Verification items for the finished model (mm, model axes). Face numbers are marked on the shaded views. A direction names the side the tool comes from. Round coordinates to 2 decimals unless told otherwise and drop trailing zeros. Write each loop counter-clockwise with the first axis right and the second up, starting at its lowest first coordinate (ties: lowest second). Pieces come first, ordered by that corner, then holes. Notation, with made-up numbers: (-25, 1.5) -> (-5, 1.5) arc R24 cw to (-5, 24.5) -> close; hole circle Ø9 at (-8, 26). An arc over 180 degrees is marked (long way). Answer as a JSON object with one key per item and string values. Group by question number.
(1) Sectioned sample at D-D on z = -8.5. Record the cut outline in (x, y).
(2) Set-up check for the marked faces 1 and 2: record each of +Z, -Z, +X, -X, +Y, -Y from which the full face is reachable in a straight line by a thin tool's end or side.
(3) Gauge pin test, flat ends, axial feed: pin 1 Ø2.5 at (x, z) = (0, -17) entering from -Y; pin 2 Ø4.5 at (x, z) = (-14.72, -8.5) entering from -Y; pin 3 Ø1.5 at (x, y) = (52.5, 1.5) entering from -Z; pin 4 Ø0.9 at (x, y) = (-53, 1.5) entering from +Z. Record the tip position at first contact, or that the pin passes through.
(4) Scan lines: L1, parallel to Z at x = -53.85, y = -1.05; L2, parallel to Z at x = 15.5, y = -1; L3, parallel to X at y = -4.6, z = 52.5. Record each from-to range of solid material in increasing order. Write a range as from..to.
(5) Sectioned sample at B-B on x = 53.85. Record the cut outline in (y, z).
(6) Sectioned sample at A-A on z = 52.5. Record the cut outline in (x, y), and give its area (3 significant figures).
(7) Sectioned sample at C-C on x = 11.5. Record the cut outline in (y, z), and give its area (3 significant figures).
```python
from build123d import *

# Parameters (mm, degrees)
SKETCH_1_W                  = 123
SKETCH_1_H                  = 130
EXTRUDE_1_DEPTH             = 5
EXTRUDE_2_DEPTH             = 3
HOLE_WIZARD_13_0_13_1_D     = 13
HOLE_WIZARD_13_0_13_1_DEPTH = 6
HOLE_WIZARD_2_5_2_5_1_D     = 2.5
HOLE_WIZARD_2_5_2_5_1_DEPTH = 5
HOLE_WIZARD_3_3_3_3_1_D     = 3.3
HOLE_WIZARD_3_3_3_3_1_DEPTH = 6
HOLE_WIZARD_1_D             = 5.2
HOLE_WIZARD_1_DEPTH         = 8
HOLE_WIZARD_1_CBORE_D       = 11
HOLE_WIZARD_1_CBORE_DEPTH   = 1
CHAMFER_1_SIZE              = 0.2
FILLET_1_R                  = 0.5
FILLET_2_R                  = 1


with BuildPart() as part:
    # 草图1 → 凸台-拉伸1 (new body)
    with BuildSketch(Plane(origin=(0, 0, 0), x_dir=(1, 0, 0), z_dir=(0, 1, 0))):
        Rectangle(SKETCH_1_W, SKETCH_1_H)
    extrude(amount=-EXTRUDE_1_DEPTH)

    # 草图2 → 凸台-拉伸2 (add)
    with BuildSketch(Plane(origin=(0, 0, 0), x_dir=(-1, 0, 0), z_dir=(0, 1, 0))):
        with BuildLine():
            Line((46.2, -45), (46.2, -60))
            Line((46.2, -60), (-46.2, -60))
            Line((-46.2, -60), (-46.2, -45))
            ThreePointArc((-46.2, -45), (-46.7, -44.5), (-47.2, -45))
            Line((-47.2, -45), (-60, -45))
            Line((-60, -45), (-60, 45))
            Line((-60, 45), (-47.2, 45))
            ThreePointArc((-47.2, 45), (-46.7, 44.5), (-46.2, 45))
            Line((-46.2, 45), (-46.2, 60))
            Line((-46.2, 60), (46.2, 60))
            Line((46.2, 60), (46.2, 45))
            ThreePointArc((46.2, 45), (46.7, 44.5), (47.2, 45))
            Line((47.2, 45), (60, 45))
            Line((60, 45), (60, -45))
            Line((60, -45), (47.2, -45))
            ThreePointArc((47.2, -45), (46.7, -44.5), (46.2, -45))
        make_face()
    extrude(amount=EXTRUDE_2_DEPTH)

    # Ø13.0 (13) 直径孔1
    with Locations(Plane(origin=(0, -5, 0), x_dir=(-1, 0, 0), z_dir=(0, -1, 0))):
        with Locations((0, 0)):
            Hole(HOLE_WIZARD_13_0_13_1_D / 2, depth=HOLE_WIZARD_13_0_13_1_DEPTH)

    # Ø2.5 (2.5) 直径孔1
    with Locations(Plane(origin=(0, 3, 0), x_dir=(1, 0, 0), z_dir=(0, 1, 0))):
        with Locations((-56.780566421, -41.855346711), (-11.041427483, 41.956342393), (-56.907566675, 41.837820676), (-11.168427737, -41.75982474)):
            Hole(HOLE_WIZARD_2_5_2_5_1_D / 2, depth=HOLE_WIZARD_2_5_2_5_1_DEPTH)

    # Ø3.3 (3.3) 直径孔1
    with Locations(Plane(origin=(0, -5, 0), x_dir=(-1, 0, 0), z_dir=(0, -1, 0))):
        with Locations((-14.722431864, -8.5), (-14.722431864, 8.5), (0, 17), (14.722431864, 8.5), (14.722431864, -8.5), (0, -17)):
            Hole(HOLE_WIZARD_3_3_3_3_1_D / 2, depth=HOLE_WIZARD_3_3_3_3_1_DEPTH)

    # 孔1
    with Locations(Plane(origin=(0, -5, 0), x_dir=(-1, 0, 0), z_dir=(0, -1, 0))):
        with Locations((53.85, 52.5), (-53.85, -52.5), (53.85, -52.5), (-53.85, 52.5)):
            CounterBoreHole(HOLE_WIZARD_1_D / 2, HOLE_WIZARD_1_CBORE_D / 2, HOLE_WIZARD_1_CBORE_DEPTH, depth=HOLE_WIZARD_1_DEPTH)

    # 倒角1
    chamfer_1_edges = [part.edges().sort_by_distance(p)[0] for p in [
        (0, -5, 65),
        (0, -5, -65),
    ]]
    chamfer(chamfer_1_edges, length=CHAMFER_1_SIZE)

    # 圆角1
    fillet_1_edges = [part.edges().sort_by_distance(p)[0] for p in [
        (-60, 1.5, -45),
        (-60, 1.5, 45),
        (-46.2, 1.5, 60),
        (46.2, 1.5, 60),
        (60, 1.5, 45),
        (60, 1.5, -45),
        (46.2, 1.5, -60),
        (-46.2, 1.5, -60),
    ]]
    fillet(fillet_1_edges, radius=FILLET_1_R)

    # 圆角2
    fillet_2_edges = [part.edges().sort_by_distance(p)[0] for p in [
        (-47.2, 1.5, -45),
        (-47.2, 1.5, 45),
        (47.2, 1.5, 45),
        (47.2, 1.5, -45),
    ]]
    fillet(fillet_2_edges, radius=FILLET_2_R)


solid = part.part
```
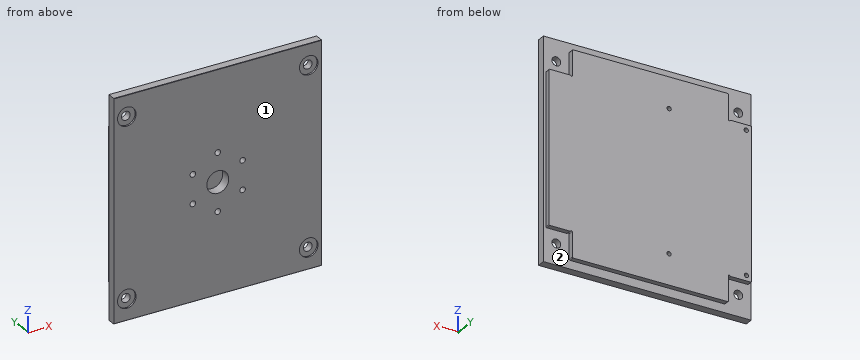
Computed values:
{
 "1": {"outline": "(-61.5, -5) -> (-16.37, -5) -> (-16.37, 1) -> (-13.07, 1) -> (-13.07, -5) -> (13.07, -5) -> (13.07, 1) -> (16.37, 1) -> (16.37, -5) -> (61.5, -5) -> (61.5, 0) -> (60, 0) -> (60, 3) -> (-60, 3) -> (-60, 0) -> (-61.5, 0) -> close"},
 "2": {"face 1": "+Z, -Z, +X, -X, -Y", "face 2": "+Y"},
 "3": {"pin 1": "y = 1", "pin 2": "y = -5", "pin 3": "z = -45", "pin 4": "z = 45"},
 "4": {"L1": "-65..-55.1, -49.9..49.9, 55.1..65", "L2": "-65..-9.96, -7.04..7.04, 9.96..65", "L3": "-61.5..-59.35, -48.35..48.35, 59.35..61.5"},
 "5": {"outline": "(-5, -64.8) -> (-4.8, -65) -> (0, -65) -> (0, -55.1) -> (-4, -55.1) -> (-4, -58) -> (-5, -58) -> close; (-5, -47) -> (-4, -47) -> (-4, -49.9) -> (0, -49.9) -> (0, -45) -> (3, -45) -> (3, 45) -> (0, 45) -> (0, 49.9) -> (-4, 49.9) -> (-4, 47) -> (-5, 47) -> close; (-5, 58) -> (-4, 58) -> (-4, 55.1) -> (0, 55.1) -> (0, 65) -> (-4.8, 65) -> (-5, 64.8) -> close"},
 "6": {"outline": "(-61.5, -5) -> (-59.35, -5) -> (-59.35, -4) -> (-56.45, -4) -> (-56.45, 0) -> (-61.5, 0) -> close; (-51.25, -4) -> (-48.35, -4) -> (-48.35, -5) -> (48.35, -5) -> (48.35, -4) -> (51.25, -4) -> (51.25, 0) -> (46.2, 0) -> (46.2, 3) -> (-46.2, 3) -> (-46.2, 0) -> (-51.25, 0) -> close; (56.45, -4) -> (59.35, -4) -> (59.35, -5) -> (61.5, -5) -> (61.5, 0) -> (56.45, 0) -> close", "area": "829 mm2"},
 "7": {"outline": "(-5, -64.8) -> (-4.8, -65) -> (0, -65) -> (0, -60) -> (3, -60) -> (3, 60) -> (0, 60) -> (0, 65) -> (-4.8, 65) -> (-5, 64.8) -> close", "area": "1,010 mm2"}
}
